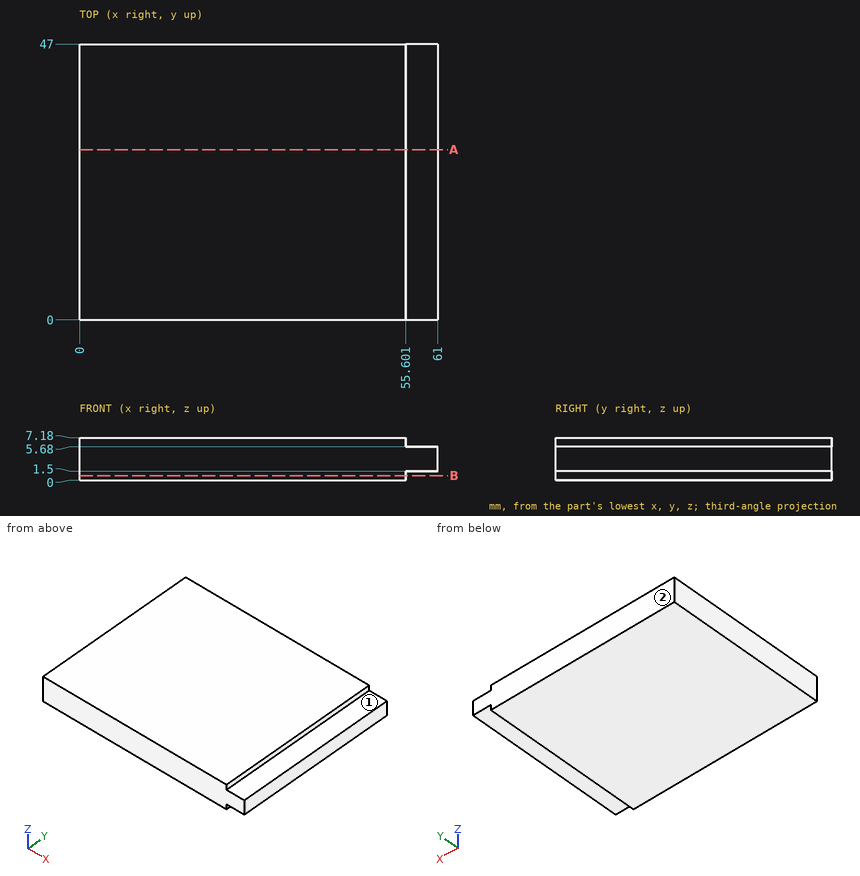
Job drawing, mm, ordinate dimensions from the low corner. One solid piece. A direction names the side the tool comes from. Give positions to 0.01 mm unless a question says otherwise; leave off trailing zeros. Loops run counter-clockwise (first coordinate to the right, second up) from the corner with the lowest first, then second, coordinate; pieces in that order, holes last. Notation, with made-up numbers: (60.25, -37) -> (112.25, -37) arc R24 cw to (112.25, -5) -> close; hole circle Ø1 at (13.5, 54.25). An arc over 180 degrees is marked (long way). Write each question's results on one line, items separated by ' | '. Start each with the question number.
Q1. Band-saw the part on B-B on z = 0.75. List the corners of the cut face in (x, y), plus the area to 3 significant figures.
Q2. Pin check, flat tips, straight feed: P1, Ø1.2, axis at y = 20, z = 0.5, coming from the +X side; P2, Ø1.6, axis at x = 58, y = 25.5, coming from the -Z side; P3, Ø1.6, axis at x = 58.5, y = 21.5, coming from the +Z side. Stop position of each tip, or through.
Q3. Which spindle directions (+Z, -Z, +X, -X, +Y, -Y) get a long thin tool onto all of the face, cutting with end or side? Do the marked faces 1 and 2. Say none if no direction does.
Q4. Band-saw the part on A-A on y = 29. List the corners of the cut face in (x, z), plus the area to 3 significant figures.
Q5. Wall check: L1, parallel to X at y = 23, z = 6.25. Give the ranges that are in metal, low to high.
Results are:
1) outline: (0, 0) -> (55.6, 0) -> (55.6, 47) -> (0, 47) -> close | area: 2,610 mm²
2) P1: stops at x = 55.6 | P2: stops at z = 1.5 | P3: stops at z = 5.68
3) face 1: +Z, +X, +Y, -Y | face 2: +Z, -Z, +X, -X, +Y
4) outline: (0, 0) -> (55.6, 0) -> (55.6, 1.5) -> (61, 1.5) -> (61, 5.68) -> (55.6, 5.68) -> (55.6, 7.18) -> (0, 7.18) -> close | area: 422 mm²
5) L1: x = 0 to 55.6
